```python
from build123d import *

# Parameters (mm, degrees)
SKETCH1_R           = 2.032
BOSS_EXTRUDE1_DEPTH = 2.54
BOSS_EXTRUDE2_START = -6.35
BOSS_EXTRUDE2_DEPTH = 6.35
BOSS_EXTRUDE3_START = 2.54
SKETCH4_R           = 2.032
BOSS_EXTRUDE3_DEPTH = 2.54
CUT_EXTRUDE2_START  = -6.35
CUT_EXTRUDE2_DEPTH  = 6.35
FILLET1_R           = 2.54
FILLET2_R           = 0.635


with BuildPart() as part:
    # Sketch1 → Boss-Extrude1 (new body)
    # profile 1 of 3: a face of its own
    with BuildSketch(Plane(origin=(0, 0, 0), x_dir=(0, 0, -1), z_dir=(1, 0, 0))):
        with BuildLine():
            Line((-6.736031019, 0), (0, 0))
            Line((0, 0), (0, 17.145))
            Line((0, 17.145), (14.2875, 17.145))
            ThreePointArc((14.2875, 17.145), (13.436761314, 20.32), (11.1125, 22.644261314))
            Line((11.1125, 22.644261314), (-12.333226749, 36.180657964))
            Line((-12.333226749, 36.180657964), (-15.422016596, 20.036703186))
            ThreePointArc((-15.422016596, 20.036703186), (-5.588466213, 12.398528792), (-6.736031019, 0))
        make_face()
    # profile 2 of 3: a face of its own
    with BuildSketch(Plane(origin=(0, 0, 0), x_dir=(0, 0, -1), z_dir=(1, 0, 0))):
        with BuildLine():
            Line((0, 0), (2.38125, 0))
            Line((2.38125, 0), (2.38125, 3.175))
            ThreePointArc((2.38125, 3.175), (3.776153955, 6.542596045), (7.14375, 7.9375))
            Line((7.14375, 7.9375), (14.2875, 7.9375))
            Line((14.2875, 7.9375), (14.2875, 17.145))
            Line((14.2875, 17.145), (0, 17.145))
            Line((0, 17.145), (0, 0))
        make_face()
        with Locations((3.175, 12.7)):
            Circle(SKETCH1_R, mode=Mode.SUBTRACT)
        with Locations((11.1125, 12.7)):
            Circle(SKETCH1_R, mode=Mode.SUBTRACT)
    # profile 3 of 3: a face of its own
    with BuildSketch(Plane(origin=(0, 0, 0), x_dir=(0, 0, -1), z_dir=(1, 0, 0))):
        with BuildLine():
            ThreePointArc((-21.168019902, 19.662272494), (-18.316086524, 20.172801019), (-15.422016596, 20.036703186))
            Line((-15.422016596, 20.036703186), (-12.333226749, 36.180657964))
            Line((-12.333226749, 36.180657964), (-43.88011314, 54.394261314))
            ThreePointArc((-43.88011314, 54.394261314), (-47.095866026, 53.827237317), (-47.095866026, 50.56187626))
            Line((-47.095866026, 50.56187626), (-21.168019902, 19.662272494))
        make_face()
    extrude(amount=BOSS_EXTRUDE1_DEPTH)

    # Sketch1<4> → Boss-Extrude2 (add)
    with BuildSketch(Plane(origin=(0, 0, 0), x_dir=(0, 0, -1), z_dir=(1, 0, 0)).offset(BOSS_EXTRUDE2_START)):
        with BuildLine():
            Line((-6.736031019, 0), (0, 0))
            Line((0, 0), (0, 17.145))
            Line((0, 17.145), (14.2875, 17.145))
            ThreePointArc((14.2875, 17.145), (13.436761314, 20.32), (11.1125, 22.644261314))
            Line((11.1125, 22.644261314), (-12.333226749, 36.180657964))
            Line((-12.333226749, 36.180657964), (-15.422016596, 20.036703186))
            ThreePointArc((-15.422016596, 20.036703186), (-5.588466213, 12.398528792), (-6.736031019, 0))
        make_face()
        with BuildLine():
            ThreePointArc((-21.168019902, 19.662272494), (-18.316086524, 20.172801019), (-15.422016596, 20.036703186))
            Line((-15.422016596, 20.036703186), (-12.333226749, 36.180657964))
            Line((-12.333226749, 36.180657964), (-43.88011314, 54.394261314))
            ThreePointArc((-43.88011314, 54.394261314), (-47.095866026, 53.827237317), (-47.095866026, 50.56187626))
            Line((-47.095866026, 50.56187626), (-21.168019902, 19.662272494))
        make_face()
    extrude(amount=BOSS_EXTRUDE2_DEPTH)

    # Sketch4 → Boss-Extrude3 (add)
    with BuildSketch(Plane.ZY.offset(6.35).offset(BOSS_EXTRUDE3_START)):
        with BuildLine():
            Line((-2.38125, 0), (6.736031019, 0))
            ThreePointArc((6.736031019, 0), (7.030863273, 14.911227359), (21.168019902, 19.662272494))
            Line((21.168019902, 19.662272494), (47.095866026, 50.56187626))
            ThreePointArc((47.095866026, 50.56187626), (47.095866026, 53.827237317), (43.88011314, 54.394261314))
            Line((43.88011314, 54.394261314), (-11.1125, 22.644261314))
            ThreePointArc((-11.1125, 22.644261314), (-13.436761314, 20.32), (-14.2875, 17.145))
            Line((-14.2875, 17.145), (-14.2875, 7.9375))
            Line((-14.2875, 7.9375), (-7.14375, 7.9375))
            ThreePointArc((-7.14375, 7.9375), (-3.776153955, 6.542596045), (-2.38125, 3.175))
            Line((-2.38125, 3.175), (-2.38125, 0))
        make_face()
        with Locations(Location((-3.175, 12.7, 0), (0, 0, 180))):
            Circle(SKETCH4_R, mode=Mode.SUBTRACT)
        with Locations(Location((-11.1125, 12.7, 0), (0, 0, 180))):
            Circle(SKETCH4_R, mode=Mode.SUBTRACT)
    extrude(amount=-BOSS_EXTRUDE3_DEPTH)

    # Sketch5 → Cut-Extrude2 (cut)
    with BuildSketch(Plane(origin=(2.54, 0, 0), x_dir=(0, 0, -1), z_dir=(1, 0, 0)).offset(CUT_EXTRUDE2_START)):
        with BuildLine():
            Line((-15.422016596, 20.036703186), (-12.333226749, 36.180657964))
            Line((-12.333226749, 36.180657964), (-43.88011314, 54.394261314))
            ThreePointArc((-43.88011314, 54.394261314), (-47.095866026, 53.827237317), (-47.095866026, 50.56187626))
            Line((-47.095866026, 50.56187626), (-21.168019902, 19.662272494))
            ThreePointArc((-21.168019902, 19.662272494), (-18.316086524, 20.172801019), (-15.422016596, 20.036703186))
        make_face()
    extrude(amount=CUT_EXTRUDE2_DEPTH, mode=Mode.SUBTRACT)

    # Fillet1
    fillet1_edges = [part.edges().sort_by_distance(p)[0] for p in [
        (-3.175, 0, 6.736031019),
        (-6.35, 19.662272494, 21.168019902),
        (-0.635, 36.180657964, 12.333226749),
        (-0.635, 20.036703186, 15.422016596),
    ]]
    fillet(fillet1_edges, radius=FILLET1_R)

    # Fillet2
    fillet2_edges = [part.edges().sort_by_distance(p)[0] for p in [
        (1.27, 7.9375, -14.2875),
        (1.27, 0, -2.38125),
        (-3.175, 17.145, -14.2875),
        (-3.175, 0, 0),
        (-7.62, 7.9375, -14.2875),
        (-7.62, 0, -2.38125),
    ]]
    fillet(fillet2_edges, radius=FILLET2_R)


solid = part.part
```
For this review, take the finished solid that the model builds, in its own axes (mm). A direction names the side the tool comes from. Round coordinates to 2 decimals unless told otherwise and drop trailing zeros. Write each loop counter-clockwise with the first axis right and the second up, starting at its lowest first coordinate (ties: lowest second). Pieces come first, ordered by that corner, then holes. Notation, with made-up numbers: (-36, -8) - (-30, -8) arc R18 cw to (-30, 1) - close; hole circle Ø3 at (9.25, 82). An arc over 180 degrees is marked (long way). Answer as CSV lines item,"result". Start each with the question number.
(1) Add section D-D, the plane z = 23. State the section outline as (x, y) points, plus the area to 3 significant figures.
(2) Add section A-A, the plane y = 12.7. State the section outline as (x, z) points, plus the area to 3 significant figures.
(3) Mouldability with a two-part tool opening along Y and no side actions: class faces 5 (the flat face through (0, 11, -5)), 6 (the cylindrical face through (-6.386, 53.789, 47.127)), 7 (the flat face through (1, 7.938, -10)), 8 (the cylindrical face through (-7.638, 14.503, -4.113)) as +Y half, -Y half, draft (parallel to the pull), parting line (faces both ways), or undercut.
(4) Machinability: for faces 1 (the flat face through (-6.35, 11, -5)), 2 (the flat face through (-8, 7.938, -10)), 3 (the cylindrical face through (-0.59, 34.49, 11.6)), 4 (the flat face through (-6.39, 35.5, 34.46)), which of the approach directions +Z, -Z, +X, -X, +Y, -Y give a long, thin tool a straight path to every point of the face, cutting with its end or side? Answer none if there is none.
(5) For pin 1 (16.5 mm diameter, centred on y = 12, z = -10.5, fed in from +X); pin 2 (1.5 mm diameter, centred on x = -7.5, y = 26, fed in from +Z); pin 3 (0.8 mm diameter, centred on x = -7, z = -10, fed in from -Y); pin 4 (10.5 mm diameter, centred on y = 32.5, z = 38, fed in from +X), all flat-tipped, find the tip position at first contact; note any pin that passes through.
(6) Add section B-B, the plane x = -7.5. State how many separate pieces and enclosed holes the cut face has, plus the area to 3 significant figures.
(7) For line 1 (Z direction, x = -8.05, y = 12.7); line 2 (X direction, y = 40.5, z = 34); line 3 (Y direction, x = 0.25, z = -3), list the stretches that pass through material, from the lowest coordinate up.
From the geometry:
1,outline,"(-8.89, 21.85) - (-3.81, 21.85) - (-3.81, 42.34) - (-8.89, 42.34) - close"
1,area,"104 mm²"
2,outline,"(-8.89, -14.29) - (-6.35, -14.29) - (-6.35, -13.14) - (-8.89, -13.14) - close; (-8.89, -9.08) - (-6.35, -9.08) - (-6.35, -5.21) - (-8.89, -5.21) - close; (-8.89, -1.14) - (-6.35, -1.14) - (-6.35, 0) - (0, 0) - (0, -1.14) - (2.54, -1.14) - (2.54, 5.72) - (-8.89, 5.72) - close; (0, -14.29) - (2.54, -14.29) - (2.54, -13.14) - (0, -13.14) - close; (0, -9.08) - (2.54, -9.08) - (2.54, -5.21) - (0, -5.21) - close"
2,area,"96.7 mm²"
3,face 5,"draft"
3,face 6,"parting line"
3,face 7,"-Y half"
3,face 8,"undercut"
4,face 1,"-Z, -Y"
4,face 2,"-Z, +X, -X, -Y"
4,face 3,"+X, +Y"
4,face 4,"+Z, +X, -X, -Y"
5,pin 1,"stops at x = 2.54"
5,pin 2,"stops at z = 27.12"
5,pin 3,"stops at y = 7.94"
5,pin 4,"stops at x = -3.81"
6,separate pieces,"1"
6,enclosed holes,"2"
6,area,"1,040 mm²"
7,line 1,"z = -14.29 to -13.14, -9.08 to -5.21, -1.14 to 5.72"
7,line 2,"x = -8.89 to -3.81"
7,line 3,"y = 5.52 to 10.68, 14.72 to 27.33"
